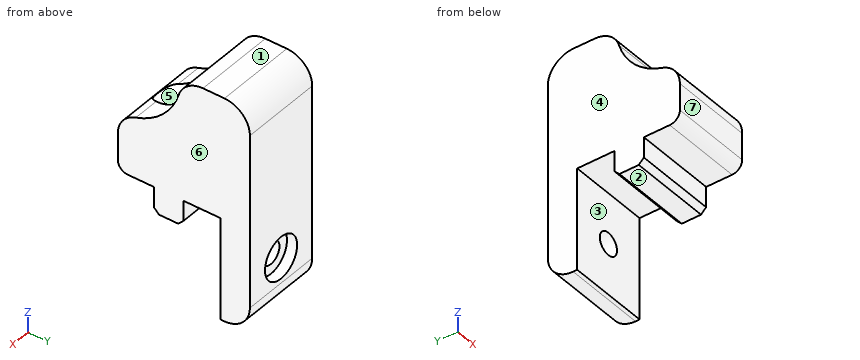
```python
from build123d import *

# Parameters (mm, degrees)
F0_W           = 16
F0_H           = 24
F1_DEPTH       = 13
F2_W           = 16
F2_H           = 5.8
F3_DEPTH       = 5
F4_DEPTH       = 20
F5_R           = 4.05
F6_DEPTH       = 20
F8_D           = 4.4
F8_CBORE_D     = 8.25
F8_CBORE_DEPTH = 2
F9_SIZE        = 1
F11_DEPTH      = 16.001
F12_T1_DEPTH   = 27.2312288127
F12_T3_DEPTH   = 27.2312288127
F12_T5_DEPTH   = 41
F12_T7_DEPTH   = 37.3525491562
F13_R          = 2


# Not quite as in the source:
# - a fillet or chamfer that OpenCascade refuses, or shapes differently, is made with other operations: its cross-section is extruded or revolved along the edge and cut away or added
# - a feature names something its author has since deleted; it is built from what else it names


with BuildPart() as f1:
    # F0 (on Front) → F1 (new body, symmetric)
    with BuildSketch(Plane.XZ):
        Rectangle(F0_W, F0_H)
    extrude(amount=F1_DEPTH, both=True)

    # F2 (on face) → F3 (join)
    with BuildSketch(Plane(origin=(0, 0, -12), x_dir=(1, 0, 0), z_dir=(0, 0, -1))):
        with Locations((0, 3)):
            Rectangle(F2_W, F2_H)
    extrude(amount=F3_DEPTH)

    # F2 (on face) → F4 (join)
    with BuildSketch(Plane(origin=(0, 0, -12), x_dir=(1, 0, 0), z_dir=(0, 0, -1))):
        with Locations((0, -10.1)):
            Rectangle(F2_W, F2_H)
    extrude(amount=F4_DEPTH)

    # F5 (on face) → F6 (cut)
    with BuildSketch(Plane.XZ.offset(13)):
        with Locations((0, 2.95)):
            Circle(F5_R)
    extrude(amount=-F6_DEPTH, mode=Mode.SUBTRACT)

    # F8 (through all)
    with Locations(Plane(origin=(0, 13, 0), x_dir=(-1, 0, 0), z_dir=(0, 1, 0))):
        with Locations((0, -22)):
            CounterBoreHole(F8_D / 2, F8_CBORE_D / 2, F8_CBORE_DEPTH)

    # F9
    f9_edges = [f1.edges().sort_by_distance(p)[0] for p in [
        (0, -5.9, -17),
        (0, -0.1, -17),
    ]]
    chamfer(f9_edges, length=F9_SIZE)

    # F10 (on face) → F11 (cut, through all)
    with BuildSketch(Plane.YZ.offset(8)):
        with BuildLine():
            Line((-13, 12), (-0.5, 12))
            ThreePointArc((-0.5, 12), (-21.8388347648, 20.8388347648), (-13, -0.5))
            Line((-13, -0.5), (-13, 12))
        make_face()
        with BuildLine():
            ThreePointArc((-13, -0.5), (-4.1611652352, 3.1611652352), (-0.5, 12))
            Line((-0.5, 12), (-13, 12))
            Line((-13, 12), (-13, -0.5))
        make_face()
    extrude(amount=-F11_DEPTH, mode=Mode.SUBTRACT)

    # F12: fillet of radius 5 on 5 edges, made by hand

    # F12_s2 → F12_t1 (cut)
    with BuildSketch(Plane.YZ.offset(-8.5549542346)):
        with BuildLine():
            ThreePointArc((-9.4285714286, 0.0210644063), (-12.0089186287, -1.7824383079), (-13, -4.7705098312))
            Line((-13, -4.7705098312), (-13, -0.5))
            ThreePointArc((-13, -0.5), (-11.1953802231, -0.369047961), (-9.4285714286, 0.0210644063))
        make_face()
    extrude(amount=F12_T1_DEPTH, mode=Mode.SUBTRACT)

    # F12_s4 → F12_t3 (cut)
    with BuildSketch(Plane.YZ.offset(-18.6762745781)):
        with BuildLine():
            ThreePointArc((-9.4285714286, 0.0210644063), (-12.0089186287, -1.7824383079), (-13, -4.7705098312))
            Line((-13, -4.7705098312), (-13, -0.5))
            ThreePointArc((-13, -0.5), (-11.1953802231, -0.369047961), (-9.4285714286, 0.0210644063))
        make_face()
    extrude(amount=F12_T3_DEPTH, mode=Mode.SUBTRACT)

    # F12_s6 → F12_t5 (cut)
    with BuildSketch(Plane.YZ.offset(-20.5)):
        with BuildLine():
            ThreePointArc((8, -32), (11.5355339059, -30.5355339059), (13, -27))
            Line((13, -27), (13, -32))
            Line((13, -32), (8, -32))
        make_face()
        with BuildLine():
            ThreePointArc((13, 7), (11.5355339059, 10.5355339059), (8, 12))
            Line((8, 12), (13, 12))
            Line((13, 12), (13, 7))
        make_face()
    extrude(amount=F12_T5_DEPTH, mode=Mode.SUBTRACT)

    # F12_s8 → F12_t7 (cut)
    with BuildSketch(Plane.YZ.offset(-18.6762745781)):
        with BuildLine():
            ThreePointArc((3.7705098312, 12), (0.7824383079, 11.0089186287), (-1.0210644063, 8.4285714286))
            ThreePointArc((-1.0210644063, 8.4285714286), (-0.630952039, 10.1953802231), (-0.5, 12))
            Line((-0.5, 12), (3.7705098312, 12))
        make_face()
    extrude(amount=F12_T7_DEPTH, mode=Mode.SUBTRACT)

    # F13
    f13_edges = [f1.edges().sort_by_distance(p)[0] for p in [
        (0, -13, -12),
    ]]
    fillet(f13_edges, radius=F13_R)


solid = f1.part
```
Build history of the part. All positions in model axes, mm. Face numbers are marked on the shaded views. A direction names the side the tool comes from. Round coordinates to 2 decimals unless told otherwise and drop trailing zeros. Write each loop counter-clockwise with the first axis right and the second up, starting at its lowest first coordinate (ties: lowest second). Pieces come first, ordered by that corner, then holes.
1) Band-saw the part on A-A, the plane z = -22. List the corners of the cut face in (x, y) (3 decimals), and give its area (3 significant figures).
2) Drill centre lines: probe 1 along X at (y, z) = (0.25, 2.95); probe 2 along Y at (x, z) = (-2.75, -21); probe 3 along Z at (x, y) = (0, -7). Where is each one in solid material? Low to high.
3) Mould opens along X. For the marked faces 4, 5, 6 and 7 say: +X half, -X half, draft (parallel to the pull), parting line (faces both ways), or undercut.
4) Pin check, flat tips, straight feed: pin 1 (1.5 mm diameter, centred on x = -6, y = 1, fed in from +Z); pin 2 (5.5 mm diameter, centred on x = 0, z = -22, fed in from +Y); pin 3 (3 mm diameter, centred on x = -5, y = 10, fed in from -Z). Stop position of each tip, or through.
5) Band-saw the part on B-B, the plane y = 4.5. List the corners of the cut face in (x, z), and give its area (3 significant figures).
6) 3-axis set-ups, long thin cutter, end or side, ignore diameter. For the marked faces 1, 2 and 3: which of +Z, -Z, +X, -X, +Y, -Y reach the whole face in a straight line?
7) Band-saw the part on D-D, the plane x = 5.75. List the corners of the cut face in (y, z), and give its area (3 significant figures).
Ans:
1. outline: (-8, 7.2) - (-2.2, 7.2) - (-2.2, 11) - (-4.125, 11) - (-4.125, 13) - (-8, 13) - close; (2.2, 7.2) - (8, 7.2) - (8, 13) - (4.125, 13) - (4.125, 11) - (2.2, 11) - close
1. area: 59.6 mm2
2. probe 1: x = -8 to -4.05, 4.05 to 8
2. probe 2: y = 7.2 to 11
2. probe 3: z = -12 to -1.1
3. face 4: -X half
3. face 5: undercut
3. face 6: +X half
3. face 7: draft
4. pin 1: stops at z = 11.57
4. pin 2: stops at y = 11
4. pin 3: stops at z = -31.97
5. outline: (-8, -12) - (8, -12) - (8, 12) - (-8, 12) - close; hole circle Ø8.1 at (0, 2.95)
5. area: 332 mm2
6. face 1: +Z, +X, -X, +Y, -Y
6. face 2: -Z, +X, -X, -Y
6. face 3: -Z, +X, -X
7. outline: (-13, -10) arc R2 ccw to (-11, -12) - (-5.9, -12) - (-5.9, -16) - (-4.9, -17) - (-1.1, -17) - (-0.1, -16) - (-0.1, -12) - (7.2, -12) - (7.2, -32) - (8, -32) arc R5 ccw to (13, -27) - (13, 7) arc R5 ccw to (8, 12) - (3.77, 12) arc R5 ccw to (-1.02, 8.43) arc R12.5 cw to (-9.43, 0.02) arc R5 ccw to (-13, -4.77) - close
7. area: 627 mm2
